Input: part model. Units: mm. Frame: model coordinates. A direction names the side the tool comes from. Coordinates: 2 decimals unless noted, no trailing zeros. Loops run counter-clockwise (first coordinate to the right, second up) from the corner with the lowest first, then second, coordinate; pieces in that order, holes last.
Item 1: Pull-direction query (Z, two-part tool) for faces 5 (the cylindrical face through (98.44, 30.21, 8.1)), 6 (the cylindrical face through (44, 30, 20)), 7 (the cylindrical face through (113.986, 29.79, 5.703)), 8 (the cylindrical face through (114.297, 29.79, 33.986)); classes: released by +Z, released by -Z, zero draft, split by the parting line, or undercut.
Item 2: Section A-A on x = 8.5. Return loops of the section in (y, z), and give its area (3 significant figures).
Item 3: Reachability of faces 1 (the flat face through (88.5, 15, 15.3)), 2 (the flat face through (15, 44, 20)), 3 (the flat face through (25, 60, 20)), 4 (the flat face through (88, 45, 15)) from +Z, -Z, +X, -X, +Y, -Y: full face, straight path, thin tool, end or side. Return the list, or none.
Item 4: Section D-D on z = 6. Return loops of the section in (x, y), and give its area (3 significant figures).
Item 5: Section B-B on z = 26.5. Return loops of the section in (x, y), and give its area (3 significant figures).
Item 6: Contact query for flat-ended pins moving along their axis: P1, Ø10, axis at x = 99, z = 26.5, coming from the +Y side; P2, Ø4, axis at x = 76, z = 30.5, coming from the -Y side; P3, Ø20, axis at x = 95.5, z = 12.5, coming from the -Y side; P4, Ø20, axis at x = 94.5, z = 26, coming from the +Y side. Output: stop coordinate, or through.
Item 7: Ray query, line 1 along Z through (x, y) = (100, 28); line 2 along Y through (x, z) = (16, 13); line 3 along Y through (x, z) = (76.5, 33). Return the intervals inside material, ascending.
Autodesk Inventor part; units mm, degrees
ref_plane "YZ Plane" through (0, 0, 0) normal (1, 0, 0) x (0, 1, 0)
ref_plane "XZ Plane" through (0, 0, 0) normal (0, 1, 0) x (-1, 0, 0)
ref_plane "XY Plane" through (0, 0, 0) normal (0, 0, 1) x (1, 0, 0)
sketch "草圖1" plane through (0, 0, 0) normal (0, 0, 1) x (1, 0, 0)
  line L0 (0, 0) -> (0, 16)
  line L1 (0, 16) -> (30, 16)
  line L2 (30, 44) -> (0, 44)
  line L3 (0, 44) -> (0, 60)
  line L4 (0, 60) -> (50, 60)
  line L5 (50, 60) -> (75.9808, 45)
  line L6 (75.9808, 45) -> (120, 45)
  line L7 (120, 45) -> (120, 15)
  line L8 (120, 15) -> (75.9808, 15)
  line L9 (75.9808, 15) -> (50, 0)
  line L10 (50, 0) -> (0, 0)
  arc A0 (30, 16) -> (30, 44) centre (30, 30) ccw
  dimension "d0" = 60
  dimension "d1" = 50
  dimension "d3" = 30
  dimension "d5" = 30
  dimension "d6" = 120
  dimension "d8" = 28
  dimension "d10" = 16
  dimension "d13" = 50
  dimension "d25" = 45
  dimension "d26" = 30
  dimension "d27" = 30
extrude "擠出1" add sketch "草圖1" along normal blind 40
fillet "圓角1" radius 20 2 edges at (120, 30, 40) (120, 30, 0)
sketch "草圖2" plane through (75.9808, 45, 40) normal (0, 1, 0) x (1, 0, 0)
  arc A0 (24.0192, 0) -> (24.0192, 40) centre (24.0192, 20) ccw
  circle A1 centre (24.0192, 20) radius 12
  point P0 (-75.9808, 40)
  dimension "d49" = 24
extrude "擠出2" cut sketch "草圖2" against normal blind 40
properties part number "複習一"
Results found:
1. face 5: undercut
1. face 6: zero draft
1. face 7: released by -Z
1. face 8: released by +Z
2. outline: (0, 0) - (16, 0) - (16, 40) - (0, 40) - close; (44, 0) - (60, 0) - (60, 40) - (44, 40) - close
2. area: 1,280 mm2
3. face 1: +Z, -Z, +X, -Y
3. face 2: +Z, -Z, -X
3. face 3: +Z, -Z, +X, -X, +Y
3. face 4: +Z, -Z, +X, +Y
4. outline: (0, 0) - (50, 0) - (75.98, 15) - (114.28, 15) - (114.28, 45) - (75.98, 45) - (50, 60) - (0, 60) - (0, 44) - (30, 44) arc R14 cw to (30, 16) - (0, 16) - close
4. area: 4,170 mm2
5. outline: (0, 0) - (50, 0) - (75.98, 15) - (89.91, 15) - (89.91, 45) - (75.98, 45) - (50, 60) - (0, 60) - (0, 44) - (30, 44) arc R14 cw to (30, 16) - (0, 16) - close; (110.09, 15) - (118.91, 15) - (118.91, 45) - (110.09, 45) - close
5. area: 3,700 mm2
6. P1: passes through
6. P2: stops at y = 13.86
6. P3: stops at y = 15
6. P4: stops at y = 45
7. line 1: z = 0 to 8, 32 to 40
7. line 2: y = 0 to 16, 44 to 60
7. line 3: y = 15 to 45
